from build123d import *

# Parameters (mm, degrees)
F0_W     = 47.625
F0_H     = 31.75
F0_R     = 2.38125
F1_DEPTH = 3.175
F2_DEPTH = 4.7625
F3_T     = -1.5875
F4_R     = 3.175
F4_R_2   = 2.38125
F5_DEPTH = 1.5875


with BuildPart() as f1:
    # F0 (on Top) → F1 (new body)
    with BuildSketch(Plane.XY):
        with Locations((7.9375, -11.90625)):
            Rectangle(F0_W, F0_H)
        with Locations((-11.90625, -23.8125)):
            Circle(F0_R, mode=Mode.SUBTRACT)
        with Locations((-3.96875, -23.8125)):
            Circle(F0_R, mode=Mode.SUBTRACT)
        with Locations((3.96875, -23.8125)):
            Circle(F0_R, mode=Mode.SUBTRACT)
        with Locations((-11.90625, -15.875)):
            Circle(F0_R, mode=Mode.SUBTRACT)
        with Locations((-3.96875, -15.875)):
            Circle(F0_R, mode=Mode.SUBTRACT)
        with Locations((3.96875, -15.875)):
            Circle(F0_R, mode=Mode.SUBTRACT)
        with Locations((11.90625, -23.8125)):
            Circle(F0_R, mode=Mode.SUBTRACT)
        with Locations((19.84375, -23.8125)):
            Circle(F0_R, mode=Mode.SUBTRACT)
        with Locations((27.78125, -23.8125)):
            Circle(F0_R, mode=Mode.SUBTRACT)
        with Locations((11.90625, -15.875)):
            Circle(F0_R, mode=Mode.SUBTRACT)
        with Locations((19.84375, -15.875)):
            Circle(F0_R, mode=Mode.SUBTRACT)
        with Locations((27.78125, -15.875)):
            Circle(F0_R, mode=Mode.SUBTRACT)
        with Locations((-11.90625, -7.9375)):
            Circle(F0_R, mode=Mode.SUBTRACT)
        with Locations((-3.96875, -7.9375)):
            Circle(F0_R, mode=Mode.SUBTRACT)
        with Locations((3.96875, -7.9375)):
            Circle(F0_R, mode=Mode.SUBTRACT)
        with Locations((-11.90625, 0)):
            Circle(F0_R, mode=Mode.SUBTRACT)
        with Locations((-3.96875, 0)):
            Circle(F0_R, mode=Mode.SUBTRACT)
        with Locations((3.96875, 0)):
            Circle(F0_R, mode=Mode.SUBTRACT)
        with Locations((11.90625, -7.9375)):
            Circle(F0_R, mode=Mode.SUBTRACT)
        with Locations((19.84375, -7.9375)):
            Circle(F0_R, mode=Mode.SUBTRACT)
        with Locations((27.78125, -7.9375)):
            Circle(F0_R, mode=Mode.SUBTRACT)
        with Locations((11.90625, 0)):
            Circle(F0_R, mode=Mode.SUBTRACT)
        with Locations((19.84375, 0)):
            Circle(F0_R, mode=Mode.SUBTRACT)
        with Locations((27.78125, 0)):
            Circle(F0_R, mode=Mode.SUBTRACT)
    extrude(amount=F1_DEPTH)

    # F0 (on Top) → F2 (join)
    with BuildSketch(Plane.XY):
        with Locations((-11.90625, 0)):
            Circle(F0_R)
        with Locations((-11.90625, -7.9375)):
            Circle(F0_R)
        with Locations((-3.96875, -7.9375)):
            Circle(F0_R)
        with Locations((-3.96875, 0)):
            Circle(F0_R)
        with Locations((3.96875, 0)):
            Circle(F0_R)
        with Locations((3.96875, -7.9375)):
            Circle(F0_R)
        with Locations((11.90625, -7.9375)):
            Circle(F0_R)
        with Locations((11.90625, 0)):
            Circle(F0_R)
        with Locations((19.84375, 0)):
            Circle(F0_R)
        with Locations((27.78125, 0)):
            Circle(F0_R)
        with Locations((27.78125, -7.9375)):
            Circle(F0_R)
        with Locations((19.84375, -7.9375)):
            Circle(F0_R)
        with Locations((-11.90625, -15.875)):
            Circle(F0_R)
        with Locations((-3.96875, -15.875)):
            Circle(F0_R)
        with Locations((3.96875, -15.875)):
            Circle(F0_R)
        with Locations((11.90625, -15.875)):
            Circle(F0_R)
        with Locations((19.84375, -15.875)):
            Circle(F0_R)
        with Locations((27.78125, -15.875)):
            Circle(F0_R)
        with Locations((27.78125, -23.8125)):
            Circle(F0_R)
        with Locations((19.84375, -23.8125)):
            Circle(F0_R)
        with Locations((11.90625, -23.8125)):
            Circle(F0_R)
        with Locations((3.96875, -23.8125)):
            Circle(F0_R)
        with Locations((-3.96875, -23.8125)):
            Circle(F0_R)
        with Locations((-11.90625, -23.8125)):
            Circle(F0_R)
    extrude(amount=F2_DEPTH)

    # F3
    f3_openings = [f1.faces().sort_by_distance(p)[0] for p in [
        (7.9375, -11.90625, 0),
    ]]
    offset(amount=F3_T, openings=f3_openings, kind=Kind.INTERSECTION)

    # F4 (on face) → F5 (join)
    with BuildSketch(Plane(origin=(0, 0, 1.5875), x_dir=(1, 0, 0), z_dir=(0, 0, -1))):
        with Locations((-7.9375, 19.84375)):
            Circle(F4_R)
        with Locations((-7.9375, 19.84375)):
            Circle(F4_R_2, mode=Mode.SUBTRACT)
        with Locations((0, 19.84375)):
            Circle(F4_R)
        with Locations((0, 19.84375)):
            Circle(F4_R_2, mode=Mode.SUBTRACT)
        with Locations((7.9375, 19.84375)):
            Circle(F4_R)
        with Locations((7.9375, 19.84375)):
            Circle(F4_R_2, mode=Mode.SUBTRACT)
        with Locations((15.875, 19.84375)):
            Circle(F4_R)
        with Locations((15.875, 19.84375)):
            Circle(F4_R_2, mode=Mode.SUBTRACT)
        with Locations((23.8125, 19.84375)):
            Circle(F4_R)
        with Locations((23.8125, 19.84375)):
            Circle(F4_R_2, mode=Mode.SUBTRACT)
        with Locations((23.8125, 11.90625)):
            Circle(F4_R)
        with Locations((23.8125, 11.90625)):
            Circle(F4_R_2, mode=Mode.SUBTRACT)
        with Locations((15.875, 11.90625)):
            Circle(F4_R)
        with Locations((15.875, 11.90625)):
            Circle(F4_R_2, mode=Mode.SUBTRACT)
        with Locations((7.9375, 11.90625)):
            Circle(F4_R)
        with Locations((7.9375, 11.90625)):
            Circle(F4_R_2, mode=Mode.SUBTRACT)
        with Locations((0, 11.90625)):
            Circle(F4_R)
        with Locations((0, 11.90625)):
            Circle(F4_R_2, mode=Mode.SUBTRACT)
        with Locations((-7.9375, 11.90625)):
            Circle(F4_R)
        with Locations((-7.9375, 11.90625)):
            Circle(F4_R_2, mode=Mode.SUBTRACT)
        with BuildLine():
            ThreePointArc((-4.7625, 3.96875), (-6.7224801022, 6.9020675157), (-10.1825640303, 6.2138140303))
            Line((-10.1825640303, 6.2138140303), (-9.6212980227, 5.6525480227))
            ThreePointArc((-9.6212980227, 5.6525480227), (-7.0262350767, 6.1687381368), (-5.55625, 3.96875))
            ThreePointArc((-5.55625, 3.96875), (-5.7375118632, 3.0574850767), (-6.2537019773, 2.2849519773))
            Line((-6.2537019773, 2.2849519773), (-5.6924359697, 1.7236859697))
            ThreePointArc((-5.6924359697, 1.7236859697), (-5.0041824843, 2.7537301022), (-4.7625, 3.96875))
        make_face()
        with BuildLine():
            Line((-9.6212980227, 5.6525480227), (-10.1825640303, 6.2138140303))
            ThreePointArc((-10.1825640303, 6.2138140303), (-10.1825640303, 1.7236859697), (-5.6924359697, 1.7236859697))
            Line((-5.6924359697, 1.7236859697), (-6.2537019773, 2.2849519773))
            ThreePointArc((-6.2537019773, 2.2849519773), (-9.6212980227, 2.2849519773), (-9.6212980227, 5.6525480227))
        make_face()
        with Locations((0, 3.96875)):
            Circle(F4_R)
        with Locations((0, 3.96875)):
            Circle(F4_R_2, mode=Mode.SUBTRACT)
        with Locations((7.9375, 3.96875)):
            Circle(F4_R)
        with Locations((7.9375, 3.96875)):
            Circle(F4_R_2, mode=Mode.SUBTRACT)
        with Locations((15.875, 3.96875)):
            Circle(F4_R)
        with Locations((15.875, 3.96875)):
            Circle(F4_R_2, mode=Mode.SUBTRACT)
        with Locations((23.8125, 3.96875)):
            Circle(F4_R)
        with Locations((23.8125, 3.96875)):
            Circle(F4_R_2, mode=Mode.SUBTRACT)
    extrude(amount=F5_DEPTH)


solid = f1.part
Could you check a few things on this model? Use its own coordinates, in mm. A direction names the side the tool comes from. Give positions to 0.01 mm unless a question says otherwise; leave off trailing zeros. Answer as a JSON object with one key per item and string values.
Q1. We'd pull the mould along Y, two halves only. Please class faces 4 (the flat face through (-12, 0, 4.762)), 5 (the cylindrical face through (18.146, -20.559, 0.805)), 6 (the cylindrical face through (25.9, -9.4, 4)): released by +Y, released by -Y, zero draft, split by the parting line, or undercut.
Taken from the geometry:
{"face 4": "zero draft", "face 5": "undercut", "face 6": "undercut"}
Q2. Which directions (+Z, -Z, +X, -X, +Y, -Y) give clear straight access to the entire face, cutting with the end or side of a thin tool? Please do faces 1 (the flat face through (4, 0, 4.762)), 2 (the flat face through (20, -24, 3.175)), 3 (the cylindrical face through (11.39, -10.262, 3.958)).
Taken from the geometry:
{"face 1": "+Z, +X, -X, +Y, -Y", "face 2": "-Z", "face 3": "+Z"}
Q3. Will these pins go through, and if not, where does the flat tip stop? pin 1 Ø3 at (x, y) = (11, -20.5) entering from +Z; pin 2 Ø3 at (x, y) = (0, -11.91) entering from +Z (3 decimals); pin 3 Ø2 at (x, y) = (-11.91, 0) entering from -Z.
Taken from the geometry:
{"pin 1": "stops at z = 4.76", "pin 2": "stops at z = 3.175", "pin 3": "stops at z = 1.59"}
Q4. Please list where these lines run through material, in increasing order: L1, parallel to Y at x = 12, z = 2.85; L2, parallel to X at y = -8, z = 3.3; L3, parallel to Y at x = -13.5, z = 4.35.
Taken from the geometry:
{"L1": "y = -27.78 to -24.6, -23.02 to -16.66, -15.09 to -8.73, -7.15 to -0.79, 0.79 to 3.97", "L2": "x = -14.29 to -9.53, -6.35 to -1.59, 1.59 to 6.35, 9.53 to 14.29, 17.46 to 22.22, 25.4 to 30.16", "L3": "y = -25.58 to -22.04, -17.64 to -14.11, -9.71 to -6.17, -1.77 to 1.77"}
